Model file for the job. Use its own axes, mm. A direction names the side the tool comes from. Give positions to 0.01 mm unless a question says otherwise; leave off trailing zeros. Loops run counter-clockwise (first coordinate to the right, second up) from the corner with the lowest first, then second, coordinate; pieces in that order, holes last. Notation, with made-up numbers: M 45,65.5 L 56,65.5 A19 cw 56,81.5 Z; hole C 75,8 d5. An arc over 180 degrees is marked long. Use CSV: the item, a comma, the result in double quotes. Start each with the question number.
(1) Wall check: line 1 along Z through (x, y) = (1.4, 0); line 2 along Z through (x, y) = (-0.6, 0). Give the ranges that are in metal, low to high. Write a range as from..to.
(2) Slice it at A-A on y = 0. List the corners of the cut face in (x, z).
(3) Slice it at B-B on z = -0.55. List the corners of the cut face in (x, y).
(4) Slice it at C-C on z = -1.4. List the corners of the cut face in (x, y), and give its area (3 significant figures).
(5) Flat gauge pins, fed straight in: P1, Ø2.5, axis at y = 0.5, z = -0.5, coming from the +X side; P2, Ø1, axis at x = 0.5, y = -1, coming from the +Z side. Where does each tip first touch, or does it go through?
(6) Two-plate mould, pull along Y, no slides. Class faces 4 (the face through (-1.5, -2, -2)), 5 (the face through (0, 0, -3)), 6 (the face through (0, 1, 0)): pulls with the +Y half, pulls with the -Y half, needs draft (parallel to the pull), parting line crosses it, or undercut.
(7) Slice it at D-D on x = -0.6. List the corners of the cut face in (y, z), and give its area (3 significant figures).
(8) Tool access for faces 1 (the face through (1.3, 0, 2)), 2 (the face through (-1.3, 0, 2)), 3 (the face through (1.5, -2, -2)): list every direction of +Z, -Z, +X, -X, +Y, -Y with a clear straight run to the whole face (end or side of a thin tool).
Autodesk Inventor part; units mm, degrees
ref_plane "YZ Plane" through (0, 0, 0) normal (1, 0, 0) x (0, 1, 0)
ref_plane "XZ Plane" through (0, 0, 0) normal (0, 1, 0) x (-1, 0, 0)
ref_plane "XY Plane" through (0, 0, 0) normal (0, 0, 1) x (1, 0, 0)
sketch "Skizze1" plane through (0, 0, 0) normal (0, 1, 0) x (-1, 0, 0)
  line L0 (1.5, 0) -> (-1.5, 0)
  line L1 (1.5, 1) -> (-1.5, 1)
  line L2 (-1.5, 1) -> (-1.5, 1.6)
  line L3 (-1.5, 1.6) -> (-1.3, 1.6)
  line L4 (-1.3, 1.6) -> (-1.3, 2.5)
  line L5 (-1.3, 2.5) -> (-1.5, 2.5)
  line L6 (-1.5, 2.5) -> (-1.5, 3)
  line L7 (-1.5, 3) -> (1.5, 3)
  line L8 (1.5, 3) -> (1.5, 2.5)
  line L9 (1.5, 2.5) -> (1.3, 2.5)
  line L10 (1.3, 2.5) -> (1.3, 1.6)
  line L11 (1.3, 1.6) -> (1.5, 1.6)
  line L12 (1.5, 1) -> (1.5, 1.6)
  line L13 (0, -0.6) -> (0, 3.6)
  point P0 (0, 0)
  dimension "d0" = 2
  dimension "d1" = 6
  dimension "d2" = 3
  dimension "d3" = 0.2
  dimension "d4" = 0.6
  dimension "d5" = 0.5
revolve "Umdrehung1" add sketch "Skizze1" angle 360 about axis through (-1.5, 0, 0) along (1, 0, 0)
equation "\"d4\" = 0.1 * d1"
properties part number "Kugellager 692-ZZ" material "Stahl, weich, geschweißt"
Reply:
1,line 1,"z = -3..-2.5, -1.6..-1, 1..1.6, 2.5..3"
1,line 2,"z = -3..-1, 1..3"
2,outline,"M -1.5,-3 L 1.5,-3 L 1.5,-2.5 L 1.3,-2.5 L 1.3,-1.6 L 1.5,-1.6 L 1.5,-1 L -1.5,-1 L -1.5,-1.6 L -1.3,-1.6 L -1.3,-2.5 L -1.5,-2.5 Z; M -1.5,1 L 1.5,1 L 1.5,1.6 L 1.3,1.6 L 1.3,2.5 L 1.5,2.5 L 1.5,3 L -1.5,3 L -1.5,2.5 L -1.3,2.5 L -1.3,1.6 L -1.5,1.6 Z"
3,outline,"M -1.5,-2.95 L 1.5,-2.95 L 1.5,-2.44 L 1.3,-2.44 L 1.3,-1.5 L 1.5,-1.5 L 1.5,-0.84 L -1.5,-0.84 L -1.5,-1.5 L -1.3,-1.5 L -1.3,-2.44 L -1.5,-2.44 Z; M -1.5,0.84 L 1.5,0.84 L 1.5,1.5 L 1.3,1.5 L 1.3,2.44 L 1.5,2.44 L 1.5,2.95 L -1.5,2.95 L -1.5,2.44 L -1.3,2.44 L -1.3,1.5 L -1.5,1.5 Z"
4,outline,"M -1.5,-2.65 L 1.5,-2.65 L 1.5,-2.07 L 1.3,-2.07 L 1.3,-0.77 L 1.5,-0.77 L 1.5,0.77 L 1.3,0.77 L 1.3,2.07 L 1.5,2.07 L 1.5,2.65 L -1.5,2.65 L -1.5,2.07 L -1.3,2.07 L -1.3,0.77 L -1.5,0.77 L -1.5,-0.77 L -1.3,-0.77 L -1.3,-2.07 L -1.5,-2.07 Z"
4,area,"14.9 mm^2"
5,P1,"stops at x = 1.5"
5,P2,"stops at z = 2.96"
6,face 4,"needs draft"
6,face 5,"parting line crosses it"
6,face 6,"undercut"
7,outline,"C 0,0 d6; hole C 0,0 d2"
7,area,"25.1 mm^2"
8,face 1,"+X"
8,face 2,"-X"
8,face 3,"+Z, -Z, +X, +Y, -Y"
